The listing builds one solid part. Answer for the finished solid, in the listing's coordinates (mm). Face numbers are marked on the shaded views. Give positions to 0.01 mm unless a question says otherwise; leave off trailing zeros. Write each loop counter-clockwise with the first axis right and the second up, starting at its lowest first coordinate (ties: lowest second). Pieces come first, ordered by that corner, then holes.
```python
from build123d import *

# Parameters (mm, degrees)
SKETCH1_R           = 5
SKETCH1_R_2         = 2.5
BOSS_EXTRUDE1_DEPTH = 4
CHAMFER1_SIZE       = 0.5
SKETCH2_R           = 4.1
SKETCH2_R_2         = 4
SKETCH2_R_3         = 3.1
SKETCH2_R_4         = 3
CUT_EXTRUDE1_DEPTH  = 0.1


with BuildPart() as part:
    # Sketch1 → Boss-Extrude1 (new body)
    with BuildSketch(Plane.XY):
        Circle(SKETCH1_R)
        Circle(SKETCH1_R_2, mode=Mode.SUBTRACT)
    extrude(amount=BOSS_EXTRUDE1_DEPTH)

    # Chamfer1
    chamfer1_edges = [part.edges().sort_by_distance(p)[0] for p in [
        (-5, 0, 0),
        (-5, 0, 4),
    ]]
    chamfer(chamfer1_edges, length=CHAMFER1_SIZE)

    # Sketch2 → Cut-Extrude1 (cut)
    # profile 1 of 2: a face of its own
    with BuildSketch(Plane(origin=(0, 0, 0), x_dir=(-1, 0, 0), z_dir=(0, 0, -1))):
        Circle(SKETCH2_R)
        Circle(SKETCH2_R_2, mode=Mode.SUBTRACT)
    # profile 2 of 2: a face of its own
    with BuildSketch(Plane(origin=(0, 0, 0), x_dir=(-1, 0, 0), z_dir=(0, 0, -1))):
        Circle(SKETCH2_R_3)
        Circle(SKETCH2_R_4, mode=Mode.SUBTRACT)
    cut_extrude1 = extrude(amount=-CUT_EXTRUDE1_DEPTH, mode=Mode.SUBTRACT)

    # Mirror1: Cut-Extrude1 across plane
    add(cut_extrude1.mirror(Plane(origin=(0, 0, 2), x_dir=(1, 0, 0), z_dir=(0, 0, -1))), mode=Mode.SUBTRACT)


solid = part.part
```
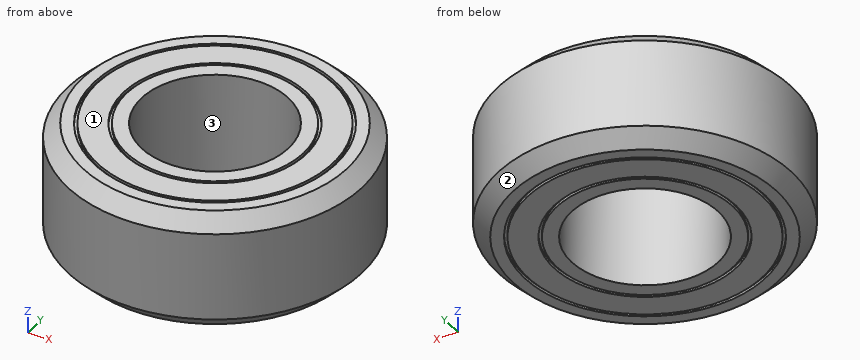
Item 1: Each of these flat-tipped pins is pushed along its axis until it touches: P1, Ø2, axis at x = -1.5, z = 2, coming from the -Y side; P2, Ø1, axis at y = 1.5, z = 1, coming from the +X side. Where does it stop, or does it pass through?
Conclusion:
P1: stops at y = -4.97
P2: stops at x = 4.9
Item 2: Determine the mould class of the marked faces 1, 2 and 3 for opening direction Y: pulls with the +Y half, pulls with the -Y half, needs draft (parallel to the pull), parting line crosses it, or undercut.
Conclusion:
face 1: needs draft
face 2: parting line crosses it
face 3: undercut
Item 3: A cutting plane is placed at A-A, the plane z = 2.25. Give the vertices of the cut face in (x, y).
Conclusion:
outline: circle Ø10 at (0, 0); hole circle Ø5 at (0, 0)
Item 4: Consider probe 1 along Y at (x, z) = (4, 2.8); probe 2 along Y at (x, z) = (3, 1.9); probe 3 along X at (y, z) = (-1.75, 2.15). Determine where each line is inside the solid, lowest interval first.
Conclusion:
probe 1: y = -3 to 3
probe 2: y = -4 to 4
probe 3: x = -4.68 to -1.79, 1.79 to 4.68
